Build history of the part. All positions in model axes, mm. A direction names the side the tool comes from. Give positions to 0.01 mm unless a question says otherwise; leave off trailing zeros. Use one line per item in the form item = value. Start each with the question number.
from build123d import *

# Parameters (mm, degrees)
SKETCH2_R                   = 79
SKETCH2_R_2                 = 24
BOSS_EXTRUDE1_DEPTH         = 3.59
BOSS_EXTRUDE2_DEPTH         = 1.5
BOSS_EXTRUDE2_DEPTH_BACK    = 5.09
SKETCH5_R                   = 48.5
SKETCH5_R_2                 = 24
CUT_EXTRUDE2_DEPTH          = 112.838759382
CUT_EXTRUDE2_DEPTH_BACK     = 112.838759382
SKETCH3_R                   = 3.75
SKETCH6_R                   = 5
CUT_EXTRUDE3_DEPTH          = 112.838759382
CHAMFER1_SIZE               = 0.75
F_1_4_0_25_DIAMETER_HOLE2_D = 6.35


with BuildPart() as part:
    # Sketch2 → Boss-Extrude1 (new body)
    with BuildSketch(Plane.XY):
        Circle(SKETCH2_R)
        Circle(SKETCH2_R_2, mode=Mode.SUBTRACT)
    extrude(amount=BOSS_EXTRUDE1_DEPTH)

    # Sketch5 → Boss-Extrude2 (add, two sides: drawn at the far end of the back side and taken through both)
    with BuildSketch(Plane.XY.offset(3.59).offset(-BOSS_EXTRUDE2_DEPTH_BACK)):
        Circle(SKETCH5_R)
        Circle(SKETCH5_R_2, mode=Mode.SUBTRACT)
    extrude(amount=BOSS_EXTRUDE2_DEPTH + BOSS_EXTRUDE2_DEPTH_BACK)

    # Sketch3 → Cut-Extrude2 (cut, two sides: drawn at the far end of the back side and taken through both)
    with BuildSketch(Plane.XY.offset(3.59).offset(-CUT_EXTRUDE2_DEPTH_BACK)):
        with Locations((0, -30)):
            Circle(SKETCH3_R)
        with Locations((-15, -25.980762114)):
            Circle(SKETCH3_R)
        with Locations((-25.980762114, -15)):
            Circle(SKETCH3_R)
        with Locations((-30, 0)):
            Circle(SKETCH3_R)
        with Locations((-25.980762114, 15)):
            Circle(SKETCH3_R)
        with Locations((-15, 25.980762114)):
            Circle(SKETCH3_R)
        with Locations((0, 30)):
            Circle(SKETCH3_R)
        with Locations((15, 25.980762114)):
            Circle(SKETCH3_R)
        with Locations((25.980762114, 15)):
            Circle(SKETCH3_R)
        with Locations((30, 0)):
            Circle(SKETCH3_R)
        with Locations((25.980762114, -15)):
            Circle(SKETCH3_R)
        with Locations((15, -25.980762114)):
            Circle(SKETCH3_R)
    extrude(amount=CUT_EXTRUDE2_DEPTH + CUT_EXTRUDE2_DEPTH_BACK, mode=Mode.SUBTRACT)

    # Sketch6 → Cut-Extrude3 (cut, through all)
    with BuildSketch(Plane.XY.offset(3.59)):
        with Locations((0, -71)):
            Circle(SKETCH6_R)
        with Locations((16, -61.451179551)):
            Circle(SKETCH6_R)
        with Locations((32, -50.494256022)):
            Circle(SKETCH6_R)
        with Locations((-61.487803669, -35.5)):
            Circle(SKETCH6_R)
        with Locations((-61.487803669, 35.5)):
            Circle(SKETCH6_R)
        with Locations((0, 71)):
            Circle(SKETCH6_R)
        with Locations((61.487803669, 35.5)):
            Circle(SKETCH6_R)
        with Locations((61.487803669, -35.5)):
            Circle(SKETCH6_R)
        with Locations((-45.218282583, -44.581996236)):
            Circle(SKETCH6_R)
        with Locations((-61.218282583, 16.869183315)):
            Circle(SKETCH6_R)
        with Locations((-16, 61.451179551)):
            Circle(SKETCH6_R)
        with Locations((45.218282583, 44.581996236)):
            Circle(SKETCH6_R)
        with Locations((61.218282583, -16.869183315)):
            Circle(SKETCH6_R)
        with Locations((-27.72930846, -52.959940932)):
            Circle(SKETCH6_R)
        with Locations((-59.72930846, -2.46568491)):
            Circle(SKETCH6_R)
        with Locations((-32, 50.494256022)):
            Circle(SKETCH6_R)
        with Locations((27.72930846, 52.959940932)):
            Circle(SKETCH6_R)
        with Locations((59.72930846, 2.46568491)):
            Circle(SKETCH6_R)
    extrude(amount=-CUT_EXTRUDE3_DEPTH, mode=Mode.SUBTRACT)

    # Chamfer1
    chamfer1_edges = [part.edges().sort_by_distance(p)[0] for p in [
        (-79, 0, 0),
        (-79, 0, 3.59),
    ]]
    chamfer(chamfer1_edges, length=CHAMFER1_SIZE)

    # 1/4 (0.25) Diameter Hole2 (through all)
    with Locations(Plane.XY.offset(5.09)):
        with Locations((27.49630657, 15.875), (0, -31.75), (-27.49630657, 15.875)):
            Hole(F_1_4_0_25_DIAMETER_HOLE2_D / 2)


solid = part.part
(1) Wall check: line 1 (X direction, y = 28.5, z = 0.75); line 2 (X direction, y = -27, z = 1.25); line 3 (Y direction, x = -12, z = 3.5). Give the ranges that are in metal, low to high. Write a range as from..to.
(2) Which spindle directions (+Z, -Z, +X, -X, +Y, -Y) get a long thin tool onto all of the face, cutting with end or side? Do faces 1 (the flat face through (34, 36, 0)), 2 (the cylindrical face through (0.066, -34.924, 1.749)). Say none if no direction does.
(3) Pin check, flat tips, straight feed: pin 1 Ø6 at (x, y) = (61.49, -35.5) entering from -Z; pin 2 Ø8.5 at (x, y) = (-15, -25.98) entering from +Z; pin 3 Ø16 at (x, y) = (-45.22, -44.58) entering from +Z; pin 4 Ø8 at (x, y) = (31, -62.5) entering from -Z. Stop position of each tip, or through.
(4) Cut at A-A, the plane x = 0. State how many separate pieces and enclosed holes the cut face has, then the cut area to 3 significant figures.
(5) Two-plate mould, pull along Y, no slides. Class faces 3 (the flat face through (34, 36, 3.59)), 4 (the cylindrical face through (-35.69, 53.87, 1.82)), 5 (the cylindrical face through (-58.23, 53.39, 1.78)): +Y half, -Y half, draft (parallel to the pull), parting line (faces both ways), or undercut.
Solution:
q1.line_1 = -73.68..-17.78, -12.22..-3.44, 3.44..12.22, 17.78..73.68
q1.line_2 = -74.24..-18.61, -11.39..-2.25, 2.25..11.39, 18.61..74.24
q1.line_3 = -77.42..-28.23, -23.73..-20.78, 20.78..23.73, 28.23..58.45, 64.45..77.42
q2.face_1 = -Z
q2.face_2 = +Z, -Z
q3.pin_1 = through
q3.pin_2 = 5.09
q3.pin_3 = 3.59
q3.pin_4 = 0
q4.separate_pieces = 6
q4.enclosed_holes = 0
q4.area = 362 mm2
q5.face_3 = draft
q5.face_4 = undercut
q5.face_5 = parting line
